```python
from build123d import *

# Parameters (mm, degrees)
BOSS_EXTRUDE1_DEPTH = 10
CHAMFER1_SIZE       = 7.802060087
CHAMFER1_SIZE_2     = 10
BOSS_EXTRUDE2_DEPTH = 20
SKETCH7_R           = 1.5
CUT_EXTRUDE1_DEPTH  = 20
CUT_EXTRUDE3_DEPTH  = 20
FILLET5_R           = 20
FILLET6_R           = 10
SKETCH10_W          = 5.3
SKETCH10_H          = 4.24
CUT_EXTRUDE4_DEPTH  = 273.805653344
SKETCH11_W          = 3.75
SKETCH11_H          = 144.691495626
CUT_EXTRUDE5_DEPTH  = 370.011076387
BOSS_EXTRUDE4_DEPTH = 12.5
SKETCH12_W          = 2
SKETCH12_H          = 1.5
CUT_EXTRUDE6_DEPTH  = 144.691496
CUT_EXTRUDE7_DEPTH  = 273.805653344
SKETCH15_W          = 8
SKETCH15_H          = 10
BOSS_EXTRUDE5_DEPTH = 8
SKETCH16_R          = 1.45
CUT_EXTRUDE9_DEPTH  = 203.44147603


with BuildPart() as part:
    # Sketch2 → Boss-Extrude1 (new, symmetric)
    with BuildSketch(Plane(origin=(0, 0, 0), x_dir=(0, 0, -1), z_dir=(1, 0, 0))):
        Polygon((36.072931518, 122.5), (-51.279924706, -117.5), (-51.279924706, -192), (-46.279924706, -192), (-46.279924706, -151.5), (-39.679924706, -151.5), (-39.679924706, -192), (-35.679924706, -192), (-35.679924706, -117.5), (-42.766502526, -117.5), (42.766502526, 117.5), (192.766502526, 117.5), (192.766502526, 122.5), align=None)
    extrude(amount=BOSS_EXTRUDE1_DEPTH, both=True)

    # Chamfer1
    # the kernel refuses this chamfer: 10, 7.802060087 mm, written as the material it adds along each edge
    with BuildSketch(Plane(origin=(-10, -117.5, 42.766502526), x_dir=(0, 0.9542611885293297, -0.298974219735734), z_dir=(1, 0, 0))) as chamfer1_piece_1_section:
        Polygon((CHAMFER1_SIZE * 0.998967402661, -CHAMFER1_SIZE * 0.0454326803806), (CHAMFER1_SIZE_2 * 0.298974219736, -CHAMFER1_SIZE_2 * 0.954261188529), (0, 0), align=None)
    chamfer1_piece_1 = extrude(amount=20, mode=Mode.PRIVATE)
    chamfer1_piece_1 = split(chamfer1_piece_1, bisect_by=Plane(origin=(0, -114.855220314, 35.679924706), z_dir=(0, 0, 1)), keep=Keep.TOP, mode=Mode.PRIVATE)
    add(chamfer1_piece_1)

    # Sketch6 → Boss-Extrude2 (add)
    with BuildSketch(Plane(origin=(10, 0, 0), x_dir=(0, 0, -1), z_dir=(1, 0, 0))):
        Polygon((-51.279924706, -180), (-66.279924706, -192), (-51.279924706, -192), align=None)
        Polygon((-35.679924706, -192), (-20.679924706, -192), (-35.679924706, -180), align=None)
    extrude(amount=-BOSS_EXTRUDE2_DEPTH)

    # Sketch7 → Cut-Extrude1 (cut)
    with BuildSketch(Plane(origin=(0, -192, 0), x_dir=(-1, 0, 0), z_dir=(0, -1, 0))):
        with Locations(Location((0, -56.279924706, 0), (0, 0, 90))):
            Circle(SKETCH7_R)
        with Locations(Location((0, -30.179924706, 0), (0, 0, 90))):
            Circle(SKETCH7_R)
    extrude(amount=-CUT_EXTRUDE1_DEPTH, mode=Mode.SUBTRACT)

    # Sketch9 → Cut-Extrude3 (cut)
    with BuildSketch(Plane(origin=(0, -187, 0), x_dir=(-1, 0, 0), z_dir=(0, -1, 0))):
        Polygon((2.75, -57.867637946), (2.75, -54.692211466), (0, -53.104498226), (-2.75, -54.692211466), (-2.75, -57.867637946), (0, -59.455351187), align=None)
        Polygon((2.75, -31.767637946), (2.75, -28.592211466), (0, -27.004498226), (-2.75, -28.592211466), (-2.75, -31.767637946), (0, -33.355351187), align=None)
    extrude(amount=-CUT_EXTRUDE3_DEPTH, mode=Mode.SUBTRACT)

    # Fillet5
    fillet5_edges = [part.edges().sort_by_distance(p)[0] for p in [
        (0, -117.5, 51.279924706),
    ]]
    fillet(fillet5_edges, radius=FILLET5_R)

    # Fillet6
    fillet6_edges = [part.edges().sort_by_distance(p)[0] for p in [
        (0, 122.5, -36.072931518),
    ]]
    fillet(fillet6_edges, radius=FILLET6_R)

    # Sketch10 → Cut-Extrude4 (cut, through all)
    with BuildSketch(Plane(origin=(10, 0, 0), x_dir=(0, 0, -1), z_dir=(1, 0, 0))):
        with Locations((-63.629924706, -189.88)):
            Rectangle(SKETCH10_W, SKETCH10_H)
        with Locations((-23.329924706, -189.88)):
            Rectangle(SKETCH10_W, SKETCH10_H)
    extrude(amount=-CUT_EXTRUDE4_DEPTH, mode=Mode.SUBTRACT)

    # Sketch11 → Cut-Extrude5 (cut, through all)
    with BuildSketch(Plane(origin=(0, 122.5, 0), x_dir=(1, 0, 0), z_dir=(0, 1, 0))):
        with Locations((-8.125, 120.420754713)):
            Rectangle(SKETCH11_W, SKETCH11_H)
        with Locations((8.125, 120.420754713)):
            Rectangle(SKETCH11_W, SKETCH11_H)
    extrude(amount=-CUT_EXTRUDE5_DEPTH, mode=Mode.SUBTRACT)

    # Sketch13 → Boss-Extrude4 (add)
    with BuildSketch(Plane(origin=(6.25, 0, 0), x_dir=(0, 0, -1), z_dir=(1, 0, 0))):
        Polygon((52.766502526, 117.5), (37.766502526, 103.762612903), (42.766502526, 117.5), align=None)
    extrude(amount=-BOSS_EXTRUDE4_DEPTH)

    # Sketch12 → Cut-Extrude6 (cut)
    with BuildSketch(Plane(origin=(0, 0, -192.766502526), x_dir=(-1, 0, 0), z_dir=(0, 0, -1))):
        with Locations((-5.25, 120)):
            Rectangle(SKETCH12_W, SKETCH12_H)
        with Locations((5.25, 120)):
            Rectangle(SKETCH12_W, SKETCH12_H)
    extrude(amount=-CUT_EXTRUDE6_DEPTH, mode=Mode.SUBTRACT)

    # Sketch14 → Cut-Extrude7 (cut, through all)
    with BuildSketch(Plane(origin=(10, 0, 0), x_dir=(0, 0, -1), z_dir=(1, 0, 0))):
        Polygon((-7.517540966, 2.736161147), (0, 0), (208.269452521, 117.586421331), (208.269452521, 129.478082523), (28.535487637, 129.478082523), align=None)
    extrude(amount=-CUT_EXTRUDE7_DEPTH, mode=Mode.SUBTRACT)

    # Sketch15 → Boss-Extrude5 (add)
    with BuildSketch(Plane(origin=(0, 2.736161147, 7.517540966), x_dir=(1, 0, 0), z_dir=(0, 0.3420201433256657, 0.9396926207859096))):
        with Locations((0, 5)):
            Rectangle(SKETCH15_W, SKETCH15_H)
    extrude(amount=-BOSS_EXTRUDE5_DEPTH)

    # Sketch16 → Cut-Extrude9 (cut, through all)
    with BuildSketch(Plane(origin=(10, 0, 0), x_dir=(0, 0, -1), z_dir=(1, 0, 0))):
        with Locations(Location((-2.048669767, 6.066543677, 0), (0, 0, 90))):
            Circle(SKETCH16_R)
    extrude(amount=-CUT_EXTRUDE9_DEPTH, mode=Mode.SUBTRACT)


solid = part.part
```
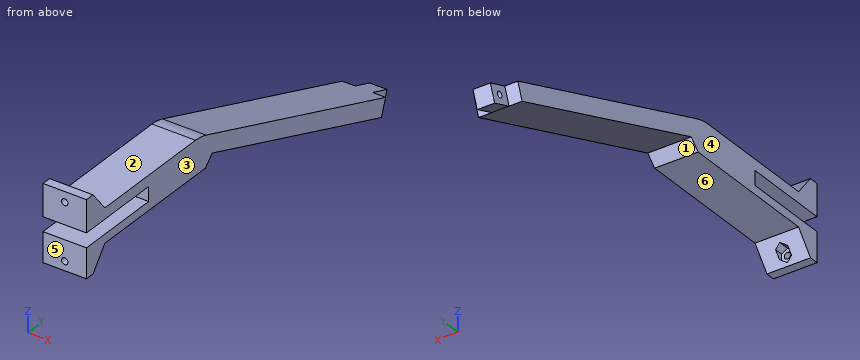
Input: part model. Units: mm. Frame: model coordinates. Face numbers are marked on the shaded views. A direction names the side the tool comes from. Give positions to 0.01 mm unless a question says otherwise; leave off trailing zeros. Order: outer loops, then holes, each group sorted by start corner. A loop starts at its lowest first (then second) coordinate and runs counter-clockwise, first axis right, second up. Notation, with made-up numbers: (41, 19) - (76, 19) arc R23 cw to (76, 48) - close; hole circle Ø11 at (-24.75, -1). An arc over 180 degrees is marked (long way). One line per item, written item: value.
1. Line query: probe 1 along Z at (x, y) = (1.5, -154.5); probe 2 along Z at (x, y) = (-3.25, -127); probe 3 along Z at (x, y) = (5.25, -88). Output: solid intervals per line, ascending.
Determined:
probe 1: 35.68 to 39.68, 46.28 to 51.28
probe 2: 35.68 to 51.28
probe 3: 32.03 to 40.54
2. Draft query along Y for the marked faces 4, 5 and 6. Return one class per face: released by +Y, released by -Y, zero draft, split by the parting line, or undercut.
Determined:
face 4: zero draft
face 5: released by -Y
face 6: undercut
3. Cut plane A-A, the plane x = 6. Output: boundary loops of the cut face in (y, z), and give its area (3 significant figures).
Determined:
outline: (-192, 25.98) - (-187.76, 25.98) - (-180, 35.68) - (-114.59, 35.68) - (-110.17, 40.1) - (0, 0) - (2.74, 7.52) - (-114.19, 50.07) arc R20 ccw to (-121.03, 51.28) - (-180, 51.28) - (-187.76, 60.98) - (-192, 60.98) - (-192, 46.28) - (-151.5, 46.28) - (-151.5, 39.68) - (-192, 39.68) - close
area: 2,100 mm2
4. Cut plane B-B, the plane y = -129.5. Output: boundary loops of the cut face in (x, z).
Determined:
outline: (-10, 35.68) - (10, 35.68) - (10, 51.28) - (-10, 51.28) - close
5. Reachability of the marked faces 1, 2 and 3 from +Z, -Z, +X, -X, +Y, -Y: full face, straight path, thin tool, end or side. Return the list, or none.
Determined:
face 1: -Z, +X, -X
face 2: +Z, +X, -X, +Y
face 3: +Z, -Z, +X, +Y, -Y
6. Pin query (flat end, axial travel): pin 1 Ø5 at (x, z) = (6.5, 25.5) entering from -Y; pin 2 Ø2.5 at (y, z) = (6.07, 2.05) entering from +X; pin 3 Ø6 at (x, y) = (0.5, -172) entering from +Z; pin 4 Ø10 at (x, y) = (3, -112.5) entering from -Z. Return the tip coordinate at first contact, or that it passes through.
Determined:
pin 1: y = -192
pin 2: through
pin 3: z = 51.28
pin 4: z = 35.68
7. Cut plane C-C, the plane z = 23.5. Output: boundary loops of the cut face in (x, y).
Determined:
outline: (-10, -64.57) - (10, -64.57) - (10, -41.18) - (-10, -41.18) - close
